The listing builds one solid part. Answer for the finished solid, in the listing's coordinates (mm). A direction names the side the tool comes from. Give positions to 0.01 mm unless a question says otherwise; leave off trailing zeros. Loops run counter-clockwise (first coordinate to the right, second up) from the corner with the lowest first, then second, coordinate; pieces in that order, holes last. Notation, with made-up numbers: (37.5, -7.5) - (91.5, -7.5) arc R28 ccw to (91.5, 17.5) - close; hole circle Ø10 at (60.25, 37). An arc over 180 degrees is marked (long way). Write item = value, one per line. Start each with the question number.
1) The part is cut by section B-B on z = 49.5. State how many separate pieces and enclosed holes the cut face has, plus the area to 3 significant figures.
2) Consider probe 1 along Y at (x, z) = (0, 103.75); probe 2 along X at (y, z) = (2, 26); probe 3 along X at (y, z) = (-0.5, 78). Determine where each line is inside the solid, lowest interval first.
3) The part is cut by section A-A on z = 4. Write down the section's boundary in (x, y), plus the area to 3 significant figures.
4) Which of the six approach directions +Z, -Z, +X, -X, +Y, -Y give full straight-line access (tool end or side, diameter ignored) to faces 4 (the flat face through (-20, 0, 7)), 5 (the cylindrical face through (0.013, -0.056, 41.043)), 6 (the flat face through (41, 0, 8))?
5) The mould has two halves that part along Y. Classify faces 1 (the flat face through (0, -6, 97)), 2 (the cylindrical face through (-30.35, 0.78, 1.52)), 3 (the cylindrical face through (0, -5, 87)): +Y half, -Y half, draft (parallel to the pull), parting line (faces both ways), or undercut.
6) Flat-ended cylindrical pins translate along their axes: P1, Ø5, axis at x = -15, z = 48.5, coming from the +Y side; P2, Ø1, axis at y = -1.5, z = 86.5, coming from the -X side; P3, Ø2.5, axis at x = -32, y = -2, coming from the +Z side. Find the tip coordinate at first contact, or state that the pin passes through.
from build123d import *

# Parameters (mm, degrees)
EXTRUDE_1_DEPTH        = 4
FILLET_1_R             = 4
SKETCH_4_R             = 2.6
CUT_EXTRUDE_1_DEPTH    = 146.708473979
FILLET_2_R             = 3
FILLET_3_R             = 3
SKETCH_6_R             = 6
EXTRUDE_3_DEPTH        = 6
CUT_EXTRUDE_2_DEPTH    = 12
FILLET_4_R             = 3
FILLET_5_R             = 2
FILLET_6_R             = 2
EXTRUDE_5_DEPTH        = 8
FILLET_7_R             = 2
FILLET_8_R             = 3
FILLET_9_R             = 2
FILLET_10_R            = 2
SKETCH_11_R            = 3
CUT_EXTRUDE_3_DEPTH    = 19
HOLE_WIZARD_M8_3_D     = 6.8
HOLE_WIZARD_M8_3_DEPTH = 15
HOLE_WIZARD_M8_3_TIP   = 2.042926105
SKETCH_14_R            = 5.6
SKETCH_14_R_2          = 2.6
EXTRUDE_6_DEPTH        = 21
EXTRUDE_START          = -21
SKETCH_15_R            = 5.6
SKETCH_15_R_2          = 2.6
EXTRUDE_7_DEPTH        = 21
FILLET_11_R            = 3


with BuildPart() as part:
    # 草图1 → 凸台-拉伸1 (new, symmetric)
    with BuildSketch(Plane(origin=(0, 0, 0), x_dir=(1, 0, 0), z_dir=(0, 1, 0))):
        with BuildLine():
            Line((-20, 0), (-41, 0))
            Line((-41, 0), (-41, -15))
            Line((-41, -15), (-55.415081473, -52.780871033))
            ThreePointArc((-55.415081473, -52.780871033), (-56.302035651, -64.020992263), (-50.968339036, -73.954707247))
            Line((-50.968339036, -73.954707247), (-17.38942166, -108))
            Line((-17.38942166, -108), (13.387176951, -108))
            add(Edge.make_bspline(
                [(11.643587669, -103.995199619), (12.175396299, -105.343239297), (12.756125427, -106.67877823), (13.387176951, -108)],
                knots=[1, 1, 1, 1, 1.048078106, 1.048078106, 1.048078106, 1.048078106], degree=3))
            add(Edge.make_bspline(
                [(29.336714137, -20), (14.953042407, -37.358957509), (2.894073745, -68.302879354), (9.112352893, -97.578972573), (11.643587669, -103.995199619)],
                knots=[0, 0, 0, 0, 0.771163971, 1, 1, 1, 1], degree=3))
            Line((29.336714137, -20), (41, -20))
            Line((41, -20), (41, -15))
            Line((41, -15), (41, 0))
            Line((41, 0), (20, 0))
            Line((20, 0), (20, -15))
            Line((20, -15), (-20, -15))
            Line((-20, -15), (-20, 0))
        make_face()
        with BuildLine():
            Line((-37.556142637, -20), (-28.778071319, -20))
            add(Edge.make_bspline(
                [(-28.778071319, -20), (-11.398449347, -43.180650425), (1.816105739, -77.326056937), (-13.829589339, -104.488932663)],
                knots=[0, 0, 0, 0, 1, 1, 1, 1], degree=3))
            Line((-13.829589339, -104.488932663), (-47.408506715, -70.44363991))
            ThreePointArc((-47.408506715, -70.44363991), (-51.408779177, -62.993353671), (-50.743563543, -54.563262749))
            Line((-50.743563543, -54.563262749), (-37.556142637, -20))
        make_face(mode=Mode.SUBTRACT)
    extrude(amount=EXTRUDE_1_DEPTH, both=True)

    # 圆角1
    fillet_1_edges = [part.edges().sort_by_distance(p)[0] for p in [
        (-30.5, 4, 0),
        (-30.5, -4, 0),
        (30.5, -4, 0),
        (30.5, 4, 0),
    ]]
    fillet(fillet_1_edges, radius=FILLET_1_R - 0.0001)  # a hair under: the kernel refuses the full size

    # 草图4 → 切除-拉伸1 (cut, through all)
    with BuildSketch(Plane(origin=(41, 0, 0), x_dir=(0, 0, -1), z_dir=(1, 0, 0))):
        with Locations((-4, 0)):
            Circle(SKETCH_4_R)
    extrude(amount=-CUT_EXTRUDE_1_DEPTH, mode=Mode.SUBTRACT)

    # 圆角2
    fillet_2_edges = [part.edges().sort_by_distance(p)[0] for p in [
        (-41, 0, 15),
        (-28.778071319, -2, 20),
        (-37.556142637, 0, 20),
        (41, 0, 20),
        (29.336714137, -2, 20),
    ]]
    fillet(fillet_2_edges, radius=FILLET_2_R)

    # 圆角3
    fillet_3_edges = [part.edges().sort_by_distance(p)[0] for p in [
        (-13.829589339, -2, 104.488932663),
    ]]
    fillet(fillet_3_edges, radius=FILLET_3_R)

    # 草图6 → 凸台-拉伸3 (add, symmetric)
    with BuildSketch(Plane(origin=(0, 0, 0), x_dir=(1, 0, 0), z_dir=(0, 1, 0))):
        with BuildLine():
            ThreePointArc((6, -93), (0, -99), (-6, -93))
            Line((-6, -93), (-6, -108))
            Line((-6, -108), (6, -108))
            Line((6, -108), (6, -93))
        make_face()
        with Locations((0, -93)):
            Circle(SKETCH_6_R)
    extrude(amount=EXTRUDE_3_DEPTH, both=True)

    # 草图9 → 切除-拉伸2 (cut)
    with BuildSketch(Plane(origin=(0, 4, 0), x_dir=(1, 0, 0), z_dir=(0, 1, 0))):
        with BuildLine():
            Line((-3.301596304, -85), (3.279031365, -85))
            add(Edge.make_bspline(
                [(23.82705745, -20.5), (19.505008519, -26.151605233), (15.701306988, -32.362525218), (9.075946345, -46.254561975), (6.412430162, -54.023271907), (3.266661612, -69.561604001), (2.686935669, -77.315763608), (3.279031365, -85)],
                knots=[0.025253164, 0.025253164, 0.025253164, 0.025253164, 0.25, 0.25, 0.5, 0.5, 0.73810851, 0.73810851, 0.73810851, 0.73810851], degree=3))
            Line((23.82705745, -20.5), (-23.464882608, -20.5))
            add(Edge.make_bspline(
                [(-23.464882608, -20.5), (-19.745298249, -25.752793711), (-16.265276937, -31.478555693), (-9.934110548, -44.200553579), (-7.185840369, -51.267285983), (-4.428907167, -62.148768173), (-3.737975942, -65.822957616), (-2.903507141, -73.212236362), (-2.760056502, -76.927560065), (-3.008657599, -82.090891991), (-3.128742658, -83.54736568), (-3.301596304, -85)],
                knots=[0.023659765, 0.023659765, 0.023659765, 0.023659765, 0.25, 0.25, 0.5, 0.5, 0.625, 0.625, 0.75, 0.75, 0.799185621, 0.799185621, 0.799185621, 0.799185621], degree=3))
        make_face()
    extrude(amount=-CUT_EXTRUDE_2_DEPTH, mode=Mode.SUBTRACT)

    # 圆角4
    fillet_4_edges = [part.edges().sort_by_distance(p)[0] for p in [
        (23.82705745, 0, 20.5),
        (-23.464882608, 0, 20.5),
    ]]
    fillet(fillet_4_edges, radius=FILLET_4_R)

    # 圆角5
    fillet_5_edges = [part.edges().sort_by_distance(p)[0] for p in [
        (-3.301596304, 0, 85),
        (3.279031365, 0, 85),
    ]]
    fillet(fillet_5_edges, radius=FILLET_5_R)

    # 圆角6
    fillet_6_edges = [part.edges().sort_by_distance(p)[0] for p in [
        (-20, 0, 15),
        (20, 0, 15),
    ]]
    fillet(fillet_6_edges, radius=FILLET_6_R)

    # 草图10 → 凸台-拉伸5 (add)
    with BuildSketch(Plane(origin=(0, 4, 0), x_dir=(1, 0, 0), z_dir=(0, 1, 0))):
        Polygon((-17.607172891, -36.773881534), (0.006004111, -45.946117812), (17.402210236, -36.768943973), (15.535837047, -33.231056027), (-0.006004111, -41.429980382), (-15.759640154, -33.226118466), align=None)
    extrude(amount=-EXTRUDE_5_DEPTH)

    # 圆角7
    fillet_7_edges = [part.edges().sort_by_distance(p)[0] for p in [
        (12.323790715, 0, 39.448007353),
        (-12.270659934, 0, 39.552923483),
    ]]
    fillet(fillet_7_edges, radius=FILLET_7_R)

    # 圆角8
    fillet_8_edges = [part.edges().sort_by_distance(p)[0] for p in [
        (-15.400235002, 0, 33.413282257),
        (15.491481072, 0, 33.254455525),
        (0.006004111, 0, 45.946117812),
        (-0.006004111, 0, 41.429980382),
    ]]
    fillet(fillet_8_edges, radius=FILLET_8_R)

    # 圆角9
    fillet_9_edges = [part.edges().sort_by_distance(p)[0] for p in [
        (13.387176951, -2, 108),
    ]]
    fillet(fillet_9_edges, radius=FILLET_9_R)

    # 圆角10
    fillet_10_edges = [part.edges().sort_by_distance(p)[0] for p in [
        (-17.38942166, 0, 108),
    ]]
    fillet(fillet_10_edges, radius=FILLET_10_R)

    # 草图11 → 切除-拉伸3 (cut)
    with BuildSketch(Plane.XY.offset(108)):
        Circle(SKETCH_11_R)
    extrude(amount=-CUT_EXTRUDE_3_DEPTH, mode=Mode.SUBTRACT)

    # M8 螺纹孔3
    with Locations(Plane.XY.offset(108)):
        with Locations((0, 0)):
            Hole(HOLE_WIZARD_M8_3_D / 2, depth=HOLE_WIZARD_M8_3_DEPTH)
            with Locations((0, 0, -(HOLE_WIZARD_M8_3_DEPTH + HOLE_WIZARD_M8_3_TIP / 2))):  # 118° drill point
                Cone(0, HOLE_WIZARD_M8_3_D / 2, HOLE_WIZARD_M8_3_TIP, mode=Mode.SUBTRACT)

    # 草图14 → 凸台-拉伸6 (add)
    with BuildSketch(Plane(origin=(41, 0, 0), x_dir=(0, 0, -1), z_dir=(1, 0, 0))):
        with Locations((-4, 0)):
            Circle(SKETCH_14_R)
        with Locations((-4, 0)):
            Circle(SKETCH_14_R_2, mode=Mode.SUBTRACT)
    extrude(amount=-EXTRUDE_6_DEPTH)

    # 草图15 → 凸台-拉伸7 (add)
    with BuildSketch(Plane.ZY.offset(41).offset(EXTRUDE_START)):
        with Locations((4, 0)):
            Circle(SKETCH_15_R)
        with Locations(Location((4, 0, 0), (0, 0, 180))):
            Circle(SKETCH_15_R_2, mode=Mode.SUBTRACT)
    extrude(amount=EXTRUDE_7_DEPTH)

    # 圆角11
    fillet_11_edges = [part.edges().sort_by_distance(p)[0] for p in [
        (30.5, -4, 7.919183588),
        (30.5, 4, 7.919183588),
        (-30.5, -4, 7.919183588),
        (-30.5, 4, 7.919183588),
    ]]
    fillet(fillet_11_edges, radius=FILLET_11_R)


solid = part.part
Answer below:
q1.separate_pieces = 3
q1.enclosed_holes = 0
q1.area = 111 mm2
q2.probe_1 = -6 to -3.4, 3.4 to 6
q2.probe_2 = -45.2 to -39.85, -24.54 to -19.77, 19.9 to 24.75
q2.probe_3 = -46.98 to -39.96, -6.87 to -2.87, 3.06 to 7.06
q3.outline = (-41, -5.6) - (-20, -5.6) - (-20, -2.6) - (-41, -2.6) - close; (-41, 2.6) - (-20, 2.6) - (-20, 5.6) - (-41, 5.6) - close; (20, -5.6) - (41, -5.6) - (41, -2.6) - (20, -2.6) - close; (20, 2.6) - (41, 2.6) - (41, 5.6) - (20, 5.6) - close
q3.area = 252 mm2
q4.face_4 = -Z, +Y, -Y
q4.face_5 = +Y, -Y
q4.face_6 = +Z, -Z, +X, +Y, -Y
q5.face_1 = -Y half
q5.face_2 = undercut
q5.face_3 = draft
q6.P1 = 4
q6.P2 = -39.09
q6.P3 = 94.45
